Read the model definition and answer for the solid it produces. Units are mm, in the model's axes. Coordinates: 2 decimals unless noted, no trailing zeros. Order: outer loops, then holes, each group sorted by start corner. A loop starts at its lowest first (then second) coordinate and runs counter-clockwise, first axis right, second up. Notation, with made-up numbers: (42.5, 53.25) -> (49.5, 53.25) arc R29 ccw to (49.5, 91.25) -> close; hole circle Ø3 at (-8.75, -27.5). An arc over 180 degrees is marked (long way). Use CSV: the item, a comma, the result in double quotes.
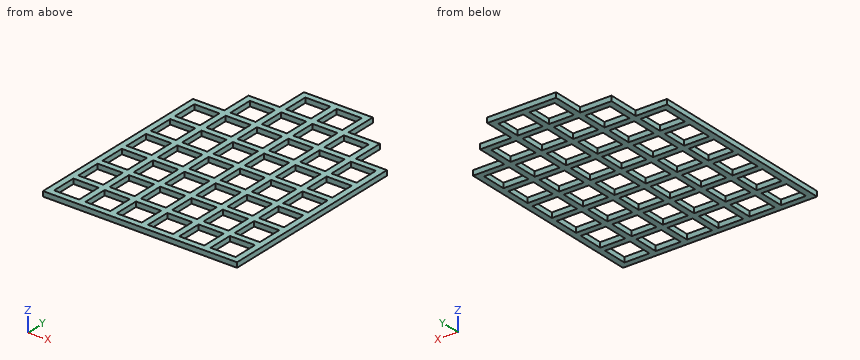
```python
from build123d import *

# Parameters (mm, degrees)
SKETCH_1_W             = 15
SKETCH_1_H             = 0.5
EXTRUDE_1_DEPTH        = 0.4
PATTERN_LINEAR_1_COUNT = 7
PATTERN_LINEAR_1_PITCH = 2.5
EXTRUDE_3_DEPTH        = 0.4
PATTERN_LINEAR_2_COUNT = 7
PATTERN_LINEAR_2_PITCH = 2.5
SKETCH_4_W             = 0.5
SKETCH_4_H             = 2.5
EXTRUDE_4_DEPTH        = 0.4
SKETCH_6_W             = 0.5
SKETCH_6_H             = 2.5
EXTRUDE_6_DEPTH        = 0.4
SKETCH_7_W             = 10.5
SKETCH_7_H             = 0.5
SKETCH_7_W_2           = 5.5
EXTRUDE_7_DEPTH        = 0.4


with BuildPart() as part:
    # Sketch 1 → Extrude 1 (new body)
    with BuildSketch(Plane.XY):
        with Locations((7.5, 0.25)):
            Rectangle(SKETCH_1_W, SKETCH_1_H)
    extrude(amount=EXTRUDE_1_DEPTH)


with BuildPart() as pattern_linear_1_1:
    # Pattern Linear 1: pattern copy
    add(part.part.moved(Location(Vector(0, 1, 0) * (1 * PATTERN_LINEAR_1_PITCH))))


with BuildPart() as pattern_linear_1_2:
    # Pattern Linear 1: pattern copy
    add(part.part.moved(Location(Vector(0, 1, 0) * (2 * PATTERN_LINEAR_1_PITCH))))


with BuildPart() as pattern_linear_1_3:
    # Pattern Linear 1: pattern copy
    add(part.part.moved(Location(Vector(0, 1, 0) * (3 * PATTERN_LINEAR_1_PITCH))))


with BuildPart() as pattern_linear_1_4:
    # Pattern Linear 1: pattern copy
    add(part.part.moved(Location(Vector(0, 1, 0) * (4 * PATTERN_LINEAR_1_PITCH))))


with BuildPart() as pattern_linear_1_5:
    # Pattern Linear 1: pattern copy
    add(part.part.moved(Location(Vector(0, 1, 0) * (5 * PATTERN_LINEAR_1_PITCH))))


with BuildPart() as pattern_linear_1_6:
    # Pattern Linear 1: pattern copy
    add(part.part.moved(Location(Vector(0, 1, 0) * (6 * PATTERN_LINEAR_1_PITCH))))


with BuildPart() as part_1:
    add(part.part)

    add(pattern_linear_1_1.part)  # Extrude 3 merges Pattern Linear 1_1

    add(pattern_linear_1_2.part)  # Extrude 3 merges Pattern Linear 1_2

    add(pattern_linear_1_3.part)  # Extrude 3 merges Pattern Linear 1_3
    # Sketch 3 → Extrude 3 (add)
    with BuildSketch(Plane.XY.offset(0.4)):
        Polygon((0, 15.5), (0, 8), (0, 0), (-0.5, 0), (-0.5, 10.98507125), (-0.5, 15.5), align=None)
    extrude_3 = extrude(amount=-EXTRUDE_3_DEPTH)

    # Pattern Linear 2: Extrude 3 ×7
    with Locations(*[(i * PATTERN_LINEAR_2_PITCH, 0, 0) for i in range(1, PATTERN_LINEAR_2_COUNT)]):
        add(extrude_3)

    add(pattern_linear_1_6.part)  # Extrude 4 merges Pattern Linear 1_6
    # Sketch 4 → Extrude 4 (add)
    with BuildSketch(Plane.XY.offset(0.4)):
        with Locations((4.75, 16.75)):
            Rectangle(SKETCH_4_W, SKETCH_4_H)
        with Locations((2.25, 16.75)):
            Rectangle(SKETCH_4_W, SKETCH_4_H)
        with Locations((7.25, 16.75)):
            Rectangle(SKETCH_4_W, SKETCH_4_H)
        with Locations((9.75, 16.75)):
            Rectangle(SKETCH_4_W, SKETCH_4_H)
        with Locations((12.25, 16.75)):
            Rectangle(SKETCH_4_W, SKETCH_4_H)
    extrude(amount=-EXTRUDE_4_DEPTH)

    # Sketch 6 → Extrude 6 (add)
    with BuildSketch(Plane.XY.offset(0.4)):
        with Locations((4.75, 19.25)):
            Rectangle(SKETCH_6_W, SKETCH_6_H)
        with Locations((9.75, 19.25)):
            Rectangle(SKETCH_6_W, SKETCH_6_H)
        with Locations((7.25, 19.25)):
            Rectangle(SKETCH_6_W, SKETCH_6_H)
    extrude(amount=-EXTRUDE_6_DEPTH)

    # Sketch 7 → Extrude 7 (add)
    with BuildSketch(Plane.XY.offset(0.4)):
        with Locations((7.25, 17.75)):
            Rectangle(SKETCH_7_W, SKETCH_7_H)
        with Locations((7.25, 20.25)):
            Rectangle(SKETCH_7_W_2, SKETCH_7_H)
    extrude(amount=-EXTRUDE_7_DEPTH)

    # Combine 1: union Pattern Linear 1_5, Pattern Linear 1_4
    add(pattern_linear_1_5.part)
    add(pattern_linear_1_4.part)


solid = part_1.part
```
Item 1: Find section D-D, the plane x = 3.25. Give the number of separate pieces and of enclosed holes in the cut face, then the cut area to 3 significant figures.
Return value:
separate pieces,"8"
enclosed holes,"0"
area,"1.60 mm^2"
Item 2: Find section B-B, the plane y = 19.25. Give the vertices of the cut face in (x, z), then the cut area to 3 significant figures.
Return value:
outline,"(4.5, 0) -> (5, 0) -> (5, 0.4) -> (4.5, 0.4) -> close; (7, 0) -> (7.5, 0) -> (7.5, 0.4) -> (7, 0.4) -> close; (9.5, 0) -> (10, 0) -> (10, 0.4) -> (9.5, 0.4) -> close"
area,"0.600 mm^2"
Item 3: Find section A-A, the plane x = 13. Give the vertices of the cut face in (y, z).
Return value:
outline,"(0, 0) -> (0.5, 0) -> (0.5, 0.4) -> (0, 0.4) -> close; (2.5, 0) -> (3, 0) -> (3, 0.4) -> (2.5, 0.4) -> close; (5, 0) -> (5.5, 0) -> (5.5, 0.4) -> (5, 0.4) -> close; (7.5, 0) -> (8, 0) -> (8, 0.4) -> (7.5, 0.4) -> close; (10, 0) -> (10.5, 0) -> (10.5, 0.4) -> (10, 0.4) -> close; (12.5, 0) -> (13, 0) -> (13, 0.4) -> (12.5, 0.4) -> close; (15, 0) -> (15.5, 0) -> (15.5, 0.4) -> (15, 0.4) -> close"
Item 4: Find section C-C, the plane y = 5.75. Give the vertices of the cut face in (x, z).
Return value:
outline,"(-0.5, 0) -> (0, 0) -> (0, 0.4) -> (-0.5, 0.4) -> close; (2, 0) -> (2.5, 0) -> (2.5, 0.4) -> (2, 0.4) -> close; (4.5, 0) -> (5, 0) -> (5, 0.4) -> (4.5, 0.4) -> close; (7, 0) -> (7.5, 0) -> (7.5, 0.4) -> (7, 0.4) -> close; (9.5, 0) -> (10, 0) -> (10, 0.4) -> (9.5, 0.4) -> close; (12, 0) -> (12.5, 0) -> (12.5, 0.4) -> (12, 0.4) -> close; (14.5, 0) -> (15, 0) -> (15, 0.4) -> (14.5, 0.4) -> close"
Item 5: This flat-tipped pin is pushed along its axis until it touches: P1, Ø4, axis at x = 3.5, y = 12, coming from the +Z side. Where does it stop, or does it pass through?
Return value:
P1,"stops at z = 0.4"
Item 6: A straight line is drawn through the part: line 1 along X through (y, z) = (19.75, 0.1). Find the intervals that lie inside material, in ascending order.
Return value:
line 1,"x = 4.5 to 5, 7 to 7.5, 9.5 to 10"
